Build history of the part. All positions in model axes, mm. A direction names the side the tool comes from. Round coordinates to 2 decimals unless told otherwise and drop trailing zeros. Write each loop counter-clockwise with the first axis right and the second up, starting at its lowest first coordinate (ties: lowest second). Pieces come first, ordered by that corner, then holes. Notation, with made-up numbers: (42.5, 8) -> (67.5, 8) arc R18 ccw to (67.5, 12) -> close; hole circle Ø2 at (11.5, -7). An arc over 180 degrees is marked (long way). Answer as CSV lines item,"result".
from build123d import *

# Parameters (mm, degrees)
SKETCH_1_W          = 300
SKETCH_1_H          = 120
SKETCH_1_R          = 48.5
EXTRUDE_1_DEPTH     = 34
FILLET_2_RADIUS     = 60
FILLET_2_LENGTH     = 34
EXTRUDE_4_DEPTH     = 10
FILLET_3_R          = 54
EXTRUDE_START       = -144
EXTRUDE_5_OUTLINE_W = 10
EXTRUDE_5_OUTLINE_H = 108
EXTRUDE_5_DEPTH     = 108
SKETCH_17_W         = 114
SKETCH_17_H         = 120
EXTRUDE_9_DEPTH     = 56
SKETCH_18_W         = 50
SKETCH_18_H         = 97
CUT_EXTRUDE_1_DEPTH = 201.089979759
SKETCH_20_R         = 29.5
CUT_EXTRUDE_2_DEPTH = 6.6
SKETCH_21_R         = 49.5
CUT_EXTRUDE_3_DEPTH = 27.7


# Read off the part's stored shape, not the designer's step: 凸台-拉伸5
with BuildPart() as part:
    # 草图1 → 凸台-拉伸1 (new body)
    with BuildSketch(Plane(origin=(0, 0, 0), x_dir=(1, 0, 0), z_dir=(0, 1, 0))):
        Rectangle(SKETCH_1_W, SKETCH_1_H)
        with Locations(Location((89.61415623, 0, 0), (0, 0, 270))):
            Circle(SKETCH_1_R, mode=Mode.SUBTRACT)
    extrude(amount=EXTRUDE_1_DEPTH)

    # 圆角2: full round fillet: the end face becomes a half cylinder, R = half its width
    fillet_2_face = Plane((150, 17, 0), x_dir=(0, -1, 0), z_dir=(1, 0, 0))  # on the end face: x along it, z out of the body
    fillet_2_slab = fillet_2_face.offset(-FILLET_2_RADIUS / 2) * Box(FILLET_2_LENGTH, 2 * FILLET_2_RADIUS, FILLET_2_RADIUS, mode=Mode.PRIVATE)  # the body's end, R deep
    fillet_2_round = Plane((90, 17, 0), x_dir=(1, 0, 0), z_dir=(0, -1, 0)) * Cylinder(FILLET_2_RADIUS, FILLET_2_LENGTH, mode=Mode.PRIVATE)  # its axis R under the face
    add(fillet_2_slab - fillet_2_round, mode=Mode.SUBTRACT)

    # 草图3 → 凸台-拉伸4 (add)
    with BuildSketch(Plane(origin=(0, 34, 0), x_dir=(1, 0, 0), z_dir=(0, 1, 0))):
        with BuildLine():
            Line((-150, -60), (90, -60))
            ThreePointArc((90, -60), (150, 0), (90, 60))
            Line((90, 60), (-150, 60))
            Line((-150, 60), (-150, -60))
        make_face()
        with BuildLine():
            Line((-144, -54), (90, -54))
            ThreePointArc((90, -54), (144, 0), (90, 54))
            Line((90, 54), (-144, 54))
            Line((-144, 54), (-144, -54))
        make_face(mode=Mode.SUBTRACT)
    extrude(amount=EXTRUDE_4_DEPTH)

    # 圆角3
    fillet_3_edges = [part.edges().sort_by_distance(p)[0] for p in [
        (-144, 39, 54),
        (-144, 39, -54),
    ]]
    fillet(fillet_3_edges, radius=FILLET_3_R - 0.0001)  # a hair under: the kernel refuses the full size

    # 凸台-拉伸5 outline → 凸台-拉伸5 (add)
    with BuildSketch(Plane.YZ.offset(EXTRUDE_START)):
        with Locations((39, 0)):
            Rectangle(EXTRUDE_5_OUTLINE_W, EXTRUDE_5_OUTLINE_H)
    extrude(amount=EXTRUDE_5_DEPTH)

    # 草图17 → 凸台-拉伸9 (add)
    with BuildSketch(Plane.XZ):
        with Locations((-93, 0)):
            Rectangle(SKETCH_17_W, SKETCH_17_H)
    extrude(amount=EXTRUDE_9_DEPTH)

    # 草图18 → 切除-拉伸1 (cut, through all)
    with BuildSketch(Plane(origin=(0, 0, -60), x_dir=(-1, 0, 0), z_dir=(0, 0, -1))):
        with Locations((91, -6)):
            Rectangle(SKETCH_18_W, SKETCH_18_H)
    extrude(amount=-CUT_EXTRUDE_1_DEPTH, mode=Mode.SUBTRACT)

    # 草图20 → 切除-拉伸2 (cut)
    with BuildSketch(Plane.ZY.offset(150)):
        with Locations((0, -6.689787926)):
            Circle(SKETCH_20_R)
    extrude(amount=-CUT_EXTRUDE_2_DEPTH, mode=Mode.SUBTRACT)

    # 草图21 → 切除-拉伸3 (cut)
    with BuildSketch(Plane.ZY.offset(143.4)):
        with Locations((0, -6.689787926)):
            Circle(SKETCH_21_R)
    extrude(amount=-CUT_EXTRUDE_3_DEPTH, mode=Mode.SUBTRACT)


solid = part.part
1. Cut at D-D, the plane y = -16. Write the cut outline in (x, z).
Results found:
outline,"(-150, -60) -> (-116, -60) -> (-116, -48.62) -> (-143.4, -48.62) -> (-143.4, -27.99) -> (-150, -27.99) -> close; (-150, 27.99) -> (-143.4, 27.99) -> (-143.4, 48.62) -> (-116, 48.62) -> (-116, 60) -> (-150, 60) -> close; (-66, -60) -> (-36, -60) -> (-36, 60) -> (-66, 60) -> close"
2. Cut at C-C, the plane x = -112. Write the cut outline in (y, z), then the cut area to 3 significant figures.
Results found:
outline,"(-56, -60) -> (-54.5, -60) -> (-54.5, 60) -> (-56, 60) -> close; (42.5, -60) -> (44, -60) -> (44, 60) -> (42.5, 60) -> close"
area,"360 mm2"
3. Which spindle directions (+Z, -Z, +X, -X, +Y, -Y) get a long thin tool onto all of the face, cutting with end or side? Do faces 1 (the flat face through (-143.4, -28, 21)), 2 (the flat face through (28, 39, -54)), 3 (the flat face through (-66, -7, -1)). Say none if no direction does.
Results found:
face 1,"none"
face 2,"+Y"
face 3,"+Z, -Z"
4. Probe line 1 along X through (y, z) = (25.5, -1); line 2 along X through (y, z) = (-2, 38); line 3 along X through (y, z) = (-36, 46). List the from-to ranges inside material, lowest first.
Results found:
line 1,"x = -150 to -143.4, -66 to 41.12, 138.1 to 149.99"
line 2,"x = -150 to -143.4, -66 to -36"
line 3,"x = -150 to -116, -66 to -36"
5. Mould opens along Z. For faces 4 (the flat face through (-94, -56, 1)), 5 (the cylindrical face through (46.586, 16.762, 22.38)), 6 (the flat face through (-32, 6, -60)) say: +Z half, -Z half, draft (parallel to the pull), parting line (faces both ways), or undercut.
Results found:
face 4,"draft"
face 5,"undercut"
face 6,"-Z half"
6. Cut at B-B, the plane y = 20. Write the cut outline in (x, z).
Results found:
outline,"(-150, -60) -> (-116, -60) -> (-116, -41.69) -> (-143.4, -41.69) -> (-143.4, -12.57) -> (-150, -12.57) -> close; (-150, 12.57) -> (-143.4, 12.57) -> (-143.4, 41.69) -> (-116, 41.69) -> (-116, 60) -> (-150, 60) -> close; (-66, -60) -> (90, -60) arc R60 ccw to (90, 60) -> (-66, 60) -> close; hole circle Ø97 at (89.61, 0)"
7. Cut at A-A, the plane z = 0. Write the cut outline in (x, y).
Results found:
outline,"(-150, -56) -> (-143.4, -56) -> (-143.4, -36.19) -> (-150, -36.19) -> close; (-150, 22.81) -> (-143.4, 22.81) -> (-143.4, 42.81) -> (-115.7, 42.81) -> (-115.7, 42.5) -> (-66, 42.5) -> (-66, -54.5) -> (-115.7, -54.5) -> (-115.7, -56) -> (-36, -56) -> (-36, 0) -> (41.11, 0) -> (41.11, 34) -> (-36, 34) -> (-36, 44) -> (-150, 44) -> close; (138.11, 0) -> (150, 0) -> (150, 44) -> (144, 44) -> (144, 34) -> (138.11, 34) -> close"
8. Drop flat-ended pins along their axis: pin 1 Ø8 at (y, z) = (40, -1) entering from +X; pin 2 Ø16.5 at (y, z) = (10, -33.5) entering from +X; pin 3 Ø10 at (y, z) = (-0.5, 38) entering from +X. Give the stop position or say it passes through.
Results found:
pin 1,"stops at x = 150"
pin 2,"stops at x = 144.43"
pin 3,"stops at x = 140.09"
